Here's the drawing with two shaded views (mm, measured from the low corner). I have some questions. A direction names the side the tool comes from. Coordinates: 2 decimals unless noted, no trailing zeros. Order: outer loops, then holes, each group sorted by start corner. A loop starts at its lowest first (then second) coordinate and runs counter-clockwise, first axis right, second up. Notation, with made-up numbers: (-29.5, 35) - (-15.5, 35) arc R23 cw to (-15.5, 56) - close; hole circle Ø6 at (15, 56.25). An arc over 180 degrees is marked (long way). Answer as a JSON object with one key per item and string values. Group by question number.
(1) Which directions (+Z, -Z, +X, -X, +Y, -Y) give clear straight access to the entire face, cutting with the end or side of a thin tool? Please do the marked faces 5, 6, 7, 8 and 9.
(2) Imagine slicing it at D-D, the plane y = 35.5. Write out the boundary of the cut face in (x, z) (1 decimal), and give its area (3 significant figures).
(3) Imagine slicing it at A-A, the plane z = 124. Write out the boundary of the cut face in (x, y).
(4) Imagine slicing it at B-B, the plane z = 256. Write out the boundary of the cut face in (x, y), and give its area (3 significant figures).
(5) We'd pull the mould along X, two halves only. Please class the marked faces 1, 2, 3 and 4: pulls with the +X half, pulls with the -X half, needs draft (parallel to the pull), parting line crosses it, or undercut.
(6) Will these pins go through, and if not, where does the flat tip stop? P1, Ø2, axis at x = 145, y = 34, coming from the -Z side; P2, Ø12, axis at y = 12, z = 255.5, coming from the -X side; P3, Ø6, axis at x = 86, y = 21.5, coming from the -Z side; P4, Ø12, axis at y = 10.5, z = 188.5, coming from the +X side.
(7) Imagine slicing it at C-C, the plane z = 163. Write out the boundary of the cut face in (x, y), and give its area (3 significant figures).
(8) Please list where these lines run through material, in increasing order: probe 1 along X at (y, z) = (19, 174); probe 2 along X at (y, z) = (9, 117.5); probe 3 along X at (y, z) = (8.5, 201.5).
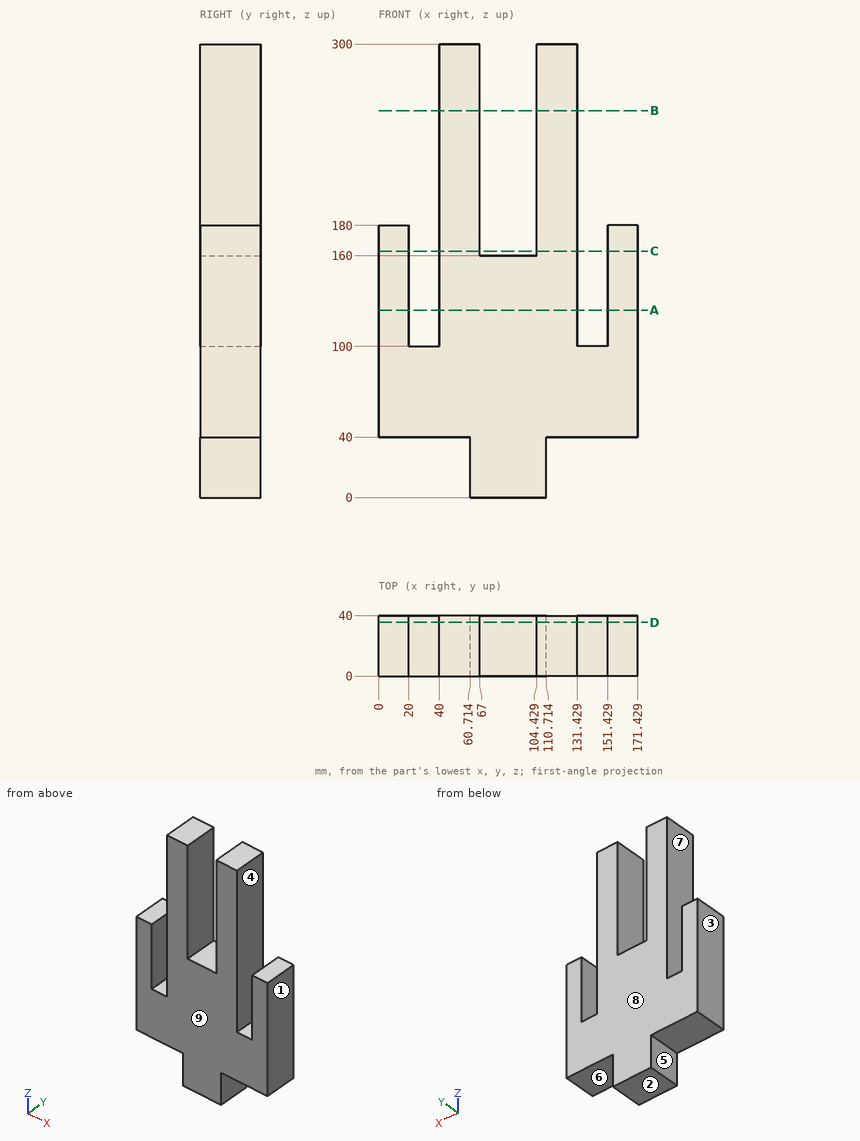
Result set:
{
 "1": {"face 5": "-Z, -X, +Y, -Y", "face 6": "-Z, +X, +Y, -Y", "face 7": "+Z, +Y, -Y", "face 8": "+Z, -Z, +X, -X, +Y", "face 9": "+Z, -Z, +X, -X, -Y"},
 "2": {"outline": "(0, 40) - (60.7, 40) - (60.7, 0) - (110.7, 0) - (110.7, 40) - (171.4, 40) - (171.4, 180) - (151.4, 180) - (151.4, 100) - (131.4, 100) - (131.4, 300) - (104.4, 300) - (104.4, 160) - (67, 160) - (67, 300) - (40, 300) - (40, 100) - (20, 100) - (20, 180) - (0, 180) - close", "area": "28,500 mm^2"},
 "3": {"outline": "(0, 0) - (20, 0) - (20, 40) - (0, 40) - close; (40, 0) - (131.43, 0) - (131.43, 40) - (40, 40) - close; (151.43, 0) - (171.43, 0) - (171.43, 40) - (151.43, 40) - close"},
 "4": {"outline": "(40, 0) - (67, 0) - (67, 40) - (40, 40) - close; (104.43, 0) - (131.43, 0) - (131.43, 40) - (104.43, 40) - close", "area": "2,160 mm^2"},
 "5": {"face 1": "pulls with the +X half", "face 2": "needs draft", "face 3": "pulls with the -X half", "face 4": "undercut"},
 "6": {"P1": "stops at z = 40", "P2": "stops at x = 40", "P3": "stops at z = 0", "P4": "stops at x = 131.43"},
 "7": {"outline": "(0, 0) - (20, 0) - (20, 40) - (0, 40) - close; (40, 0) - (67, 0) - (67, 40) - (40, 40) - close; (104.43, 0) - (131.43, 0) - (131.43, 40) - (104.43, 40) - close; (151.43, 0) - (171.43, 0) - (171.43, 40) - (151.43, 40) - close", "area": "3,760 mm^2"},
 "8": {"probe 1": "x = 0 to 20, 40 to 67, 104.43 to 131.43, 151.43 to 171.43", "probe 2": "x = 0 to 20, 40 to 131.43, 151.43 to 171.43", "probe 3": "x = 40 to 67, 104.43 to 131.43"}
}
